For this review, take the finished solid that the model builds, in its own axes (mm). A direction names the side the tool comes from. Give positions to 0.01 mm unless a question says otherwise; leave off trailing zeros. Write each loop counter-clockwise with the first axis right and the second up, starting at its lowest first coordinate (ties: lowest second). Pieces come first, ordered by that corner, then holes.
1) We need section A-A on y = 6.35. Give the boundary of the cut face in (x, z) (3 decimals), and give its area (3 significant figures).
2) Draft analysis for pull direction Y (two halves, no side actions). For faces 1 (the face through (85.73, 6.49, -16.43)), 2 (the face through (51, 0, -17)), 3 (the face through (0, 6, -28)), state which applies: pulls with the +Y half, pulls with the -Y half, needs draft (parallel to the pull), parting line crosses it, or undercut.
3) We need section C-C on z = -15. Give the boundary of the cut face in (x, y) (3 decimals), and give its area (3 significant figures).
4) For P1, Ø6.5, axis at x = -14.5, y = 4.5, coming from the +Z side; P2, Ø3, axis at y = 4.5, z = -28, coming from the -X side; P3, Ø6.5, axis at x = -19, y = 7.5, coming from the -Z side; P4, Ø1.5, axis at x = 70, z = -11, coming from the -Y side, all flat-tipped, find the tip position at first contact; note any pin that passes through.
5) Machinability: for faces 4 (the face through (-25.4, 6, -17)), 5 (the face through (-13, 6, -10.315)), 6 (the face through (-13, 6, -23.015)), which of the approach directions +Z, -Z, +X, -X, +Y, -Y give a long, thin tool a straight path to every point of the face, cutting with its end or side? Answer none if there is none.
6) We need section D-D on x = -11. Give the boundary of the cut face in (y, z), and give its area (3 significant figures).
7) Wall thickness on line 1 along Y through (x, z) = (88.9, -16) (3 decimals); line 2 along X through (y, z) = (6.5, -8); line 3 along X through (y, z) = (11.25, -5): over which ranges is each line inside the solid? List them lowest first.
8) We need section B-B on x = 88.9. Give the boundary of the cut face in (y, z) (3 decimals).
from build123d import *

# Parameters (mm, degrees)
SKETCH1_W           = 101.6
SKETCH1_H           = 33.330801688
BOSS_EXTRUDE1_DEPTH = 12.7
SKETCH2_W           = 12.7
SKETCH2_H           = 12.7
BOSS_EXTRUDE2_DEPTH = 25.4
SKETCH4_R           = 3.175
CUT_EXTRUDE2_DEPTH  = 108.679117479


with BuildPart() as part:
    # Sketch1 → Boss-Extrude1 (new body)
    with BuildSketch(Plane(origin=(0, 0, 0), x_dir=(1, 0, 0), z_dir=(0, 1, 0))):
        with Locations((50.8, 16.665400844)):
            Rectangle(SKETCH1_W, SKETCH1_H)
    extrude(amount=BOSS_EXTRUDE1_DEPTH)

    # Sketch2 → Boss-Extrude2 (add)
    with BuildSketch(Plane.ZY):
        with Locations((-16.665400844, 6.35)):
            Rectangle(SKETCH2_W, SKETCH2_H)
    extrude(amount=BOSS_EXTRUDE2_DEPTH)

    # Sketch4 → Cut-Extrude2 (cut, through all)
    with BuildSketch(Plane.XY):
        with Locations((88.9, 6.35)):
            Circle(SKETCH4_R)
    extrude(amount=-CUT_EXTRUDE2_DEPTH, mode=Mode.SUBTRACT)


solid = part.part
Results list:
1. outline: (-25.4, -23.015) - (0, -23.015) - (0, -33.331) - (85.725, -33.331) - (85.725, 0) - (0, 0) - (0, -10.315) - (-25.4, -10.315) - close; (92.075, -33.331) - (101.6, -33.331) - (101.6, 0) - (92.075, 0) - close
1. area: 3,500 mm2
2. face 1: undercut
2. face 2: pulls with the -Y half
2. face 3: needs draft
3. outline: (-25.4, 0) - (101.6, 0) - (101.6, 12.7) - (-25.4, 12.7) - close; hole circle Ø6.35 at (88.9, 6.35)
3. area: 1,580 mm2
4. P1: stops at z = -10.32
4. P2: stops at x = 0
4. P3: stops at z = -23.02
4. P4: stops at y = 0
5. face 4: +Z, -Z, -X, +Y, -Y
5. face 5: +Z, -X, +Y, -Y
5. face 6: -Z, -X, +Y, -Y
6. outline: (0, -23.02) - (12.7, -23.02) - (12.7, -10.32) - (0, -10.32) - close
6. area: 161 mm2
7. line 1: y = 0 to 3.175, 9.525 to 12.7
7. line 2: x = 0 to 85.73, 92.07 to 101.6
7. line 3: x = 0 to 101.6
8. outline: (0, -33.331) - (3.175, -33.331) - (3.175, 0) - (0, 0) - close; (9.525, -33.331) - (12.7, -33.331) - (12.7, 0) - (9.525, 0) - close
